Geometry check sheet. Reference: the model listing, model coordinates, mm. A direction names the side the tool comes from. Coordinates: 2 decimals unless noted, no trailing zeros. Order: outer loops, then holes, each group sorted by start corner. A loop starts at its lowest first (then second) coordinate and runs counter-clockwise, first axis right, second up. Notation, with made-up numbers: (61.5, 57.5) - (116.5, 57.5) arc R24 ccw to (116.5, 78.5) - close; hole circle Ø9 at (-34, 16). An arc over 180 degrees is marked (long way). Put each result on its own line as item: value.
from build123d import *

# Parameters (mm, degrees)
SKETCH1_W               = 132
SKETCH1_H               = 72
BOSS_EXTRUDE1_DEPTH     = 47.625
CUT_EXTRUDE1_DEPTH      = 1
CUT_EXTRUDE1_DEPTH_BACK = 96.25
SKETCH3_W               = 96
SKETCH3_H               = 38.1
CUT_EXTRUDE2_DEPTH      = 73
SKETCH4_R               = 15
CUT_EXTRUDE3_DEPTH      = 133
SKETCH5_R               = 36
SKETCH5_R_2             = 15
BOSS_EXTRUDE2_DEPTH     = 16
SKETCH6_R               = 12
CUT_EXTRUDE4_DEPTH      = 96.25


with BuildPart() as part:
    # Sketch1 → Boss-Extrude1 (new body, symmetric)
    with BuildSketch(Plane.XY):
        Rectangle(SKETCH1_W, SKETCH1_H)
    extrude(amount=BOSS_EXTRUDE1_DEPTH, both=True)

    # Sketch2 → Cut-Extrude1 (cut, two sides)
    with BuildSketch(Plane.XY.offset(47.625)) as cut_extrude1_sk:
        with BuildLine():
            Line((220.000004886, 36), (-30, 36))
            ThreePointArc((-30, 36), (-66, 1.527e-06), (-30.000003054, -36))
            Line((-30.000003054, -36), (220.000001832, -36.000021206))
            Line((220.000001832, -36.000021206), (-280.000007939, -36))
            Line((-280.000007939, -36), (-280.000004886, 36.000021206))
            Line((-280.000004886, 36.000021206), (220.000004886, 36))
        make_face()
    extrude(amount=CUT_EXTRUDE1_DEPTH, mode=Mode.SUBTRACT)
    extrude(cut_extrude1_sk.sketch, amount=-CUT_EXTRUDE1_DEPTH_BACK, mode=Mode.SUBTRACT)

    # Sketch3 → Cut-Extrude2 (cut, through all)
    with BuildSketch(Plane(origin=(0, 36, 0), x_dir=(1, 0, 0), z_dir=(0, 1, 0))):
        with Locations((-18, 0)):
            Rectangle(SKETCH3_W, SKETCH3_H)
    extrude(amount=-CUT_EXTRUDE2_DEPTH, mode=Mode.SUBTRACT)

    # Sketch4 → Cut-Extrude3 (cut, through all)
    with BuildSketch(Plane(origin=(66, 0, 0), x_dir=(0, 0, -1), z_dir=(1, 0, 0))):
        Circle(SKETCH4_R)
    extrude(amount=-CUT_EXTRUDE3_DEPTH, mode=Mode.SUBTRACT)

    # Sketch5 → Boss-Extrude2 (add)
    with BuildSketch(Plane(origin=(66, 0, 0), x_dir=(0, 0, -1), z_dir=(1, 0, 0))):
        Circle(SKETCH5_R)
        Circle(SKETCH5_R_2, mode=Mode.SUBTRACT)
    extrude(amount=BOSS_EXTRUDE2_DEPTH)

    # Sketch6 → Cut-Extrude4 (cut, through all)
    with BuildSketch(Plane.XY.offset(47.625)):
        with Locations((-30, 0)):
            Circle(SKETCH6_R)
    extrude(amount=-CUT_EXTRUDE4_DEPTH, mode=Mode.SUBTRACT)


solid = part.part
Q1. Section check A-A on y = 0. Record the boundary of the cut face in (x, z) (3 decimals), then the cut area to 3 significant figures.
Answer block:
outline: (-66, -47.625) - (-42, -47.625) - (-42, -19.05) - (-66, -19.05) - close; (-66, 19.05) - (-42, 19.05) - (-42, 47.625) - (-66, 47.625) - close; (-18, -47.625) - (66, -47.625) - (66, -36) - (82, -36) - (82, -15) - (30, -15) - (30, -19.05) - (-18, -19.05) - close; (-18, 19.05) - (30, 19.05) - (30, 15) - (82, 15) - (82, 36) - (66, 36) - (66, 47.625) - (-18, 47.625) - close
area: 7,140 mm^2
Q2. Section check B-B on x = 10. Record the boundary of the cut face in (y, z) (3 decimals).
Answer block:
outline: (-36, -47.625) - (36, -47.625) - (36, -19.05) - (-36, -19.05) - close; (-36, 19.05) - (36, 19.05) - (36, 47.625) - (-36, 47.625) - close
Q3. Thickness scan on L1, parallel to Y at x = 39.5, z = 0; L2, parallel to Z at x = -8.5, y = -32.5 (3 decimals); L3, parallel to Y at x = -30, z = 32. Record the ranges inside material, lowest first. Write a range as [from, to].
Answer block:
L1: y = [-36, -15], [15, 36]
L2: z = [-47.625, -19.05], [19.05, 47.625]
L3: y = [-36, -12], [12, 36]
Q4. Section check C-C on z = 41. Record the boundary of the cut face in (x, y), then the cut area to 3 significant figures.
Answer block:
outline: (-30, -36) - (66, -36) - (66, 36) - (-30, 36) arc R36 ccw to start; hole circle Ø24 at (-30, 0)
area: 8,500 mm^2
Q5. Access from +Z, -Z, +X, -X, +Y, -Y to the whole of each face (thin tool, end or side, straight path). Record for faces 5 (the cylindrical face through (73.888, 35.694, 4.686)), 6 (the flat face through (-8, 1, -19.05)), 7 (the flat face through (66, -1, -39)), 8 (the flat face through (66, -1, 40)), 9 (the flat face through (82, -15.5, 0.5)).
Answer block:
face 5: +X
face 6: -X, +Y, -Y
face 7: -Z, +X
face 8: +Z, +X
face 9: +Z, -Z, +X, +Y, -Y
Q6. Draft check along X on faces 1 (the cylindrical face through (-65.99, 0.79, -33.14)), 2 (the cylindrical face through (-18.915, -4.596, 33.538)), 3 (the flat face through (-1, 1, 47.625)), 4 (the cylindrical face through (-18.915, -4.596, -33.137)). Enter one of: pulls with the +X half, pulls with the -X half, needs draft (parallel to the pull), parting line crosses it, or undercut.
Answer block:
face 1: pulls with the -X half
face 2: undercut
face 3: needs draft
face 4: undercut
Q7. Depth check by flat-ended pin: pin 1 Ø2 at (y, z) = (23, 31) entering from +X. Enter the tip coordinate at first touch or a pass-through.
Answer block:
pin 1: stops at x = 66
Q8. Section check D-D on z = -10.5. Record the boundary of the cut face in (x, y), then the cut area to 3 significant figures.
Answer block:
outline: (30, -36) - (66, -36) - (66, -34.43) - (82, -34.43) - (82, -10.71) - (30, -10.71) - close; (30, 10.71) - (82, 10.71) - (82, 34.43) - (66, 34.43) - (66, 36) - (30, 36) - close
area: 2,580 mm^2
